The figure shows three views and two pictorial views of one solid part (mm, origin at its lowest corner). Answer the questions. A direction names the side the tool comes from. Round coordinates to 2 decimals unless told otherwise and drop trailing zeros. Order: outer loops, then holes, each group sorted by start corner. A loop starts at its lowest first (then second) coordinate and runs counter-clockwise, first axis right, second up. Notation, with made-up numbers: (-21, 56) - (7, 56) arc R25 cw to (7, 88) - close; hole circle Ø5 at (40.25, 78). An arc over 180 degrees is marked (long way). Use CSV: the item, a comma, the result in double quotes.
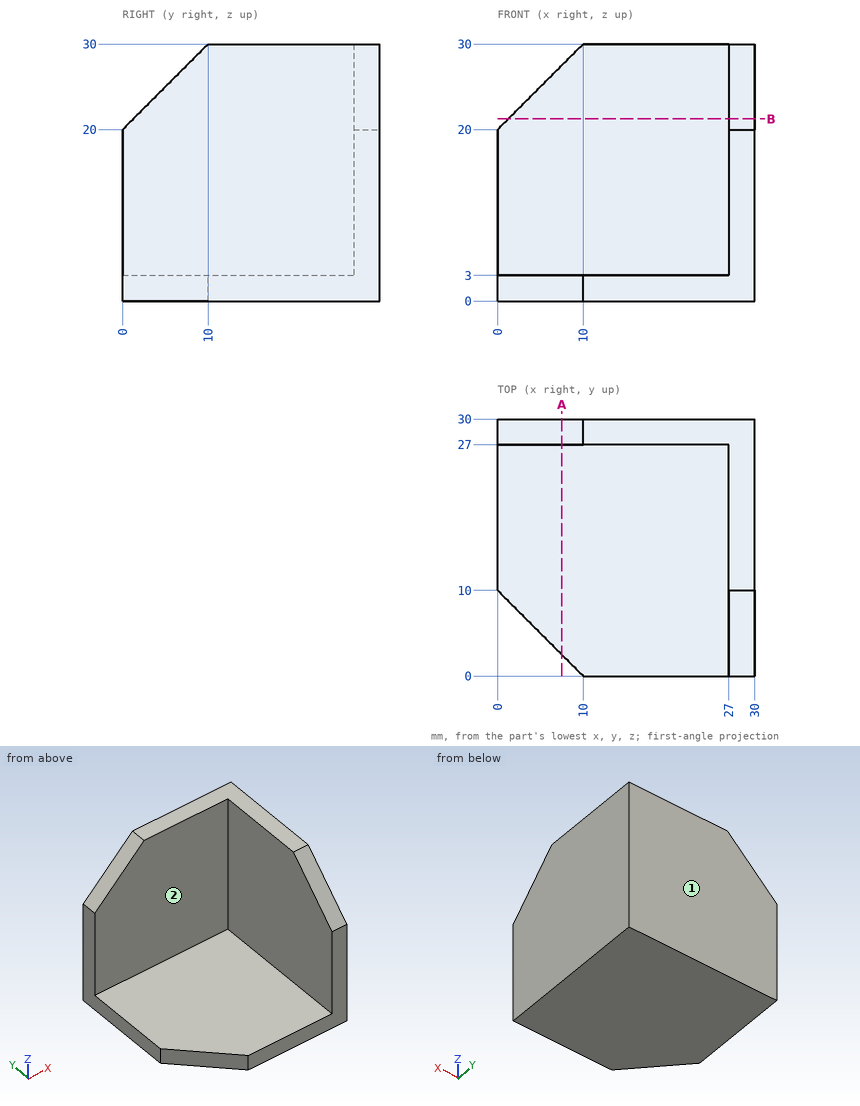
(1) Find section B-B (z = 21.25). Determine the outline of the cut face in (x, y), and give its area (4 significant figures).
Findings below:
outline,"(1.25, 27) - (27, 27) - (27, 1.25) - (30, 1.25) - (30, 30) - (1.25, 30) - close"
area,"163.5 mm²"
(2) Find the intervals of material crossed by L1, parallel to X at y = 12.75, z = 16.75; L2, parallel to Z at x = 2.5, y = 22.25, in increasing order. Write a range as from..to.
Findings below:
L1,"x = 27..30"
L2,"z = 0..3"
(3) Find section A-A (x = 7.5). Determine the outline of the cut face in (y, z).
Findings below:
outline,"(2.5, 0) - (30, 0) - (30, 27.5) - (27, 27.5) - (27, 3) - (2.5, 3) - close"
(4) Each of these flat-tipped pins is pushed along its axis until it touches: pin 1 (1.5 mm diameter, centred on x = 4.5, z = 24.5, fed in from -Y); pin 2 (12 mm diameter, centred on y = 16.5, z = 17.5, fed in from -X); pin 3 (8 mm diameter, centred on x = 7.5, y = 19.5, fed in from +Z). Where does it stop, or does it pass through?
Findings below:
pin 1,"stops at y = 27"
pin 2,"stops at x = 27"
pin 3,"stops at z = 3"
(5) For the marked faces 1 and 2, determine the directions among +Z, -Z, +X, -X, +Y, -Y from which every point of the face is accessible in a straight line to the end or side of a thin tool.
Findings below:
face 1,"+Z, -Z, +X, -X, +Y"
face 2,"+Z, -X, -Y"
